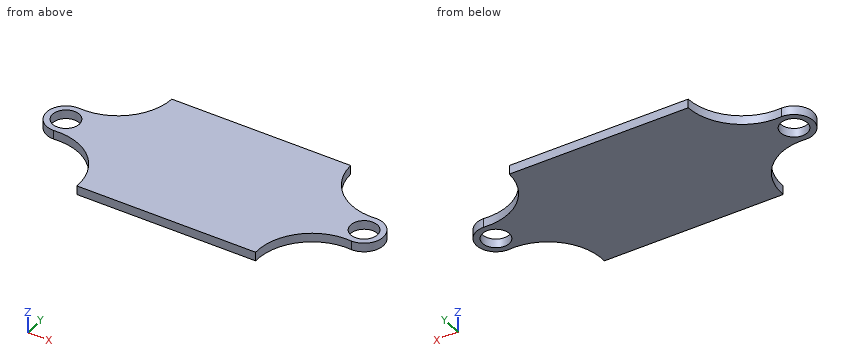
```python
from build123d import *

# Parameters (mm, degrees)
SKETCH2_R           = 4.5
BOSS_EXTRUDE2_DEPTH = 3


with BuildPart() as part:
    # Sketch2 → Boss-Extrude2 (new body)
    with BuildSketch(Plane.XY):
        with BuildLine():
            ThreePointArc((-50, -5.834500909), (-56.5, 0.665499091), (-50, 7.165499091))
            ThreePointArc((-50, 7.165499091), (-36.130190824, 11.743060763), (-30, 25))
            Line((-30, 25), (30, 25))
            ThreePointArc((30, 25), (36.130190824, 11.743060763), (50, 7.165499091))
            ThreePointArc((50, 7.165499091), (56.5, 0.665499091), (50, -5.834500909))
            ThreePointArc((50, -5.834500909), (35.63018968, -10.857170595), (30, -25))
            Line((30, -25), (-30, -25))
            ThreePointArc((-30, -25), (-35.63018968, -10.857170595), (-50, -5.834500909))
        make_face()
        with Locations((50, 0.665499091)):
            Circle(SKETCH2_R, mode=Mode.SUBTRACT)
        with Locations((-50, 0.665499091)):
            Circle(SKETCH2_R, mode=Mode.SUBTRACT)
    extrude(amount=BOSS_EXTRUDE2_DEPTH)


solid = part.part
```
Model file for the job. Use its own axes, mm. Coordinates: 2 decimals unless noted, no trailing zeros. Write each loop counter-clockwise with the first axis right and the second up, starting at its lowest first coordinate (ties: lowest second). Pieces come first, ordered by that corner, then holes. Notation, with made-up numbers: (-24, 46) - (17, 46) arc R26 ccw to (17, 82) - close; hole circle Ø11 at (60, 41.5). An arc over 180 degrees is marked (long way). Use a Markdown table: item, result. Add a question column.
Item 1: Drill centre lines: line 1 along Y through (x, z) = (-50, 2.1); line 2 along X through (y, z) = (-0.5, 2.85); line 3 along X through (y, z) = (-2.5, 1.9). Where is each one in solid material? Low to high.
Item 2: Band-saw the part on A-A, the plane z = 2. Write the cut outline in (x, y), and give its area (3 significant figures).
Item 3: Drop flat-ended pins along their axis: pin 1 (1 mm diameter, centred on y = 16.5, z = 1.5, fed in from -X); pin 2 (10.5 mm diameter, centred on x = 50, y = 0.67, fed in from -Z); pin 3 (1 mm diameter, centred on x = -41, z = 1.5, fed in from +Y). Give the stop position or say it passes through.
Item 4: Band-saw the part on C-C, the plane y = -20. Write the cut outline in (x, z).
Item 5: Band-saw the part on B-B, the plane x = 44. Write the cut outline in (y, z), and give its area (3 significant figures).
A:
| question | item | result |
|---|---|---|
| 1 | line 1 | y = -5.83 to -3.83, 5.17 to 7.17 |
| 1 | line 2 | x = -56.39 to -54.35, -45.65 to 45.65, 54.35 to 56.39 |
| 1 | line 3 | x = -55.68 to -53.2, -46.8 to 46.8, 53.2 to 55.68 |
| 2 | outline | (-50, -5.83) arc R18.34 cw to (-30, -25) - (30, -25) arc R18.34 cw to (50, -5.83) arc R6.5 ccw to (50, 7.17) arc R18.34 cw to (30, 25) - (-30, 25) arc R18.34 cw to (-50, 7.17) arc R6.5 ccw to start; hole circle Ø9 at (-50, 0.67); hole circle Ø9 at (50, 0.67) |
| 2 | area | 3,810 mm² |
| 3 | pin 1 | stops at x = -32.61 |
| 3 | pin 2 | stops at z = 0 |
| 3 | pin 3 | stops at y = 8.85 |
| 4 | outline | (-30.44, 0) - (30.44, 0) - (30.44, 3) - (-30.44, 3) - close |
| 5 | outline | (-6.27, 0) - (7.61, 0) - (7.61, 3) - (-6.27, 3) - close |
| 5 | area | 41.7 mm² |
